```python
from build123d import *

# Parameters (mm, degrees)
F0_R     = 9
F1_DEPTH = 4
F3_W     = 3
F3_H     = 3
F4_DEPTH = 2
F2_R     = 9
F2_R_2   = 8
F5_DEPTH = 1


# Not quite as in the source:
# - a feature names something its author has since deleted; it is built from what else it names


with BuildPart() as f1:
    # F0 (on Top) → F1 (new body)
    with BuildSketch(Plane.XY):
        with Locations((-31.3306450844, 19.7580661625)):
            Circle(F0_R)
    extrude(amount=F1_DEPTH)

    # F3 (on face) → F4 (cut)
    with BuildSketch(Plane(origin=(0, 0, 0), x_dir=(1, 0, 0), z_dir=(0, 0, -1))):
        with BuildLine():
            ThreePointArc((-32.8306450844, -28.6321858371), (-32.0832814269, -28.7265408676), (-31.3306450844, -28.7580661625))
            ThreePointArc((-31.3306450844, -28.7580661625), (-30.5780087419, -28.7265408676), (-29.8306450844, -28.6321858371))
            Line((-29.8306450844, -28.6321858371), (-29.8306450844, -21.2580661625))
            Line((-29.8306450844, -21.2580661625), (-32.8306450844, -21.2580661625))
            Line((-32.8306450844, -21.2580661625), (-32.8306450844, -28.6321858371))
        make_face()
        with BuildLine():
            ThreePointArc((-40.204764759, -18.2580661625), (-40.2991197895, -19.0054298199), (-40.3306450844, -19.7580661625))
            ThreePointArc((-40.3306450844, -19.7580661625), (-40.2991197895, -20.510702505), (-40.204764759, -21.2580661625))
            Line((-40.204764759, -21.2580661625), (-32.8306450844, -21.2580661625))
            Line((-32.8306450844, -21.2580661625), (-32.8306450844, -18.2580661625))
            Line((-32.8306450844, -18.2580661625), (-40.204764759, -18.2580661625))
        make_face()
        with Locations((-31.3306450844, -19.7580661625)):
            Rectangle(F3_W, F3_H)
        with BuildLine():
            Line((-29.8306450844, -18.2580661625), (-29.8306450844, -21.2580661625))
            Line((-29.8306450844, -21.2580661625), (-22.4565254097, -21.2580661625))
            ThreePointArc((-22.4565254097, -21.2580661625), (-22.3621703793, -20.510702505), (-22.3306450844, -19.7580661625))
            ThreePointArc((-22.3306450844, -19.7580661625), (-22.3621703793, -19.0054298199), (-22.4565254097, -18.2580661625))
            Line((-22.4565254097, -18.2580661625), (-29.8306450844, -18.2580661625))
        make_face()
        with BuildLine():
            Line((-32.8306450844, -10.8839464878), (-32.8306450844, -18.2580661625))
            Line((-32.8306450844, -18.2580661625), (-29.8306450844, -18.2580661625))
            Line((-29.8306450844, -18.2580661625), (-29.8306450844, -10.8839464878))
            ThreePointArc((-29.8306450844, -10.8839464878), (-30.5780087419, -10.7895914574), (-31.3306450844, -10.7580661625))
            ThreePointArc((-31.3306450844, -10.7580661625), (-32.0832814269, -10.7895914574), (-32.8306450844, -10.8839464878))
        make_face()
    extrude(amount=-F4_DEPTH, mode=Mode.SUBTRACT)

    # F2 (on face) → F5 (join)
    with BuildSketch(Plane.XY.offset(4)):
        with Locations((-31.3306450844, 19.7580661625)):
            Circle(F2_R)
        with Locations((-31.3306450844, 19.7580661625)):
            Circle(F2_R_2, mode=Mode.SUBTRACT)
    extrude(amount=F5_DEPTH)


solid = f1.part
```
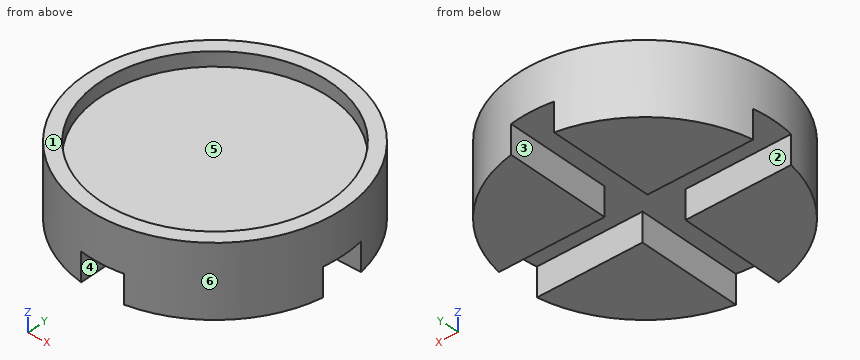
Geometry check sheet. Reference: the model listing, model coordinates, mm. Face numbers are marked on the shaded views. A direction names the side the tool comes from. Give positions to 0.01 mm unless a question says otherwise; leave off trailing zeros. Write each loop counter-clockwise with the first axis right and the second up, starting at its lowest first coordinate (ties: lowest second). Pieces come first, ordered by that corner, then holes.
1) Gauge pin test, flat ends, axial feed: pin 1 (1 mm diameter, centred on x = -27.5, z = 1, fed in from -Y); pin 2 (0.6 mm diameter, centred on y = 23.5, z = 1, fed in from -X); pin 3 (1.6 mm diameter, centred on y = 23.5, z = 1, fed in from +X). Record the tip position at first contact, or that the pin passes through.
2) Access from +Z, -Z, +X, -X, +Y, -Y to the whole of each face (thin tool, end or side, straight path). Record for the marked faces 1, 2 and 3.
3) Section check D-D, the plane z = 4.3. Record the boundary of the cut face in (x, y), and give its area (3 significant figures).
4) Release check for a two-part mould opening along Y. For the marked faces 4, 5 and 6 record: pulls with the +Y half, pulls with the -Y half, needs draft (parallel to the pull), parting line crosses it, or undercut.
5) Material ranges on L1, parallel to X at y = 19.5, z = 3.5; L2, parallel to Z at x = -33.25, y = 20.5; L3, parallel to Y at x = -28.25, z = 0.7, recorded low to high.
6) Section check C-C, the plane x = -29.25. Record the boundary of the cut face in (y, z).
7) Section check A-A, the plane z = 0.65. Record the boundary of the cut face in (x, y).
8) Section check B-B, the plane y = 24.75. Record the boundary of the cut face in (x, z), and give its area (3 significant figures).
Computed:
1. pin 1: stops at y = 11.4
1. pin 2: stops at x = -39.65
1. pin 3: stops at x = -22.83
2. face 1: +Z, +X, -X, +Y, -Y
2. face 2: -Z, +X, -X
2. face 3: -Z, +Y, -Y
3. outline: circle Ø18 at (-31.33, 19.76); hole circle Ø16 at (-31.33, 19.76)
3. area: 53.4 mm2
4. face 4: needs draft
4. face 5: undercut
4. face 6: parting line crosses it
5. L1: x = -40.33 to -22.33
5. L2: z = 2 to 4
5. L3: y = 11.3 to 18.26, 21.26 to 28.21
6. outline: (11, 0) - (18.26, 0) - (18.26, 2) - (21.26, 2) - (21.26, 0) - (28.51, 0) - (28.51, 5) - (27.48, 5) - (27.48, 4) - (12.03, 4) - (12.03, 5) - (11, 5) - close
7. outline: (-40.2, 18.26) arc R9 ccw to (-32.83, 10.88) - (-32.83, 18.26) - close; (-40.2, 21.26) - (-32.83, 21.26) - (-32.83, 28.63) arc R9 ccw to start; (-29.83, 10.88) arc R9 ccw to (-22.46, 18.26) - (-29.83, 18.26) - close; (-29.83, 21.26) - (-22.46, 21.26) arc R9 ccw to (-29.83, 28.63) - close
8. outline: (-38.82, 0) - (-32.83, 0) - (-32.83, 2) - (-29.83, 2) - (-29.83, 0) - (-23.84, 0) - (-23.84, 5) - (-25.08, 5) - (-25.08, 4) - (-37.58, 4) - (-37.58, 5) - (-38.82, 5) - close
8. area: 56.4 mm2
